Geometry check sheet. Reference: the model listing, model coordinates, mm. Face numbers are marked on the shaded views. A direction names the side the tool comes from. Coordinates: 2 decimals unless noted, no trailing zeros. Write each loop counter-clockwise with the first axis right and the second up, starting at its lowest first coordinate (ties: lowest second). Pieces come first, ordered by that corner, then holes. Notation, with made-up numbers: (32, 1) -> (67, 1) arc R23 ccw to (67, 27) -> close; hole circle Ø10 at (39.25, 41.5). An arc over 180 degrees is marked (long way). Answer in a Markdown table with one row per item. Add a question column.
1. Cross-section at A-A on y = 56.5. Record the cut outline in (x, z).
2. Cross-section at D-D on x = 14. Record the cut outline in (y, z).
3. Depth check by flat-ended pin: P1, Ø8, axis at y = 50, z = -22.5, coming from the +X side; P2, Ø1.5, axis at y = 59, z = -21.5, coming from the +X side; P3, Ø2.5, axis at y = 65.04, z = -23.5, coming from the +X side. Enter the tip coordinate at first touch or a pass-through.
4. Mould release check, pull along Y, two halves, no side actions. Record for the marked faces 1, 2 and 3: pulls with the +Y half, pulls with the -Y half, needs draft (parallel to the pull), parting line crosses it, or undercut.
5. Scan lines: L1, parallel to Y at x = 6.5, z = -29.5; L2, parallel to Y at x = 14, z = -20.25; L3, parallel to Y at x = 16.5, z = -29.75. Record each from-to range of solid material in increasing order. Write a range as from..to.
6. Set-up check for the marked faces 4, 5 and 6: record each of +Z, -Z, +X, -X, +Y, -Y from which the full face is reachable in a straight line by a thin tool's end or side.
7. Cross-section at C-C on z = -30.25. Record the cut outline in (x, y), and give its area (3 significant figures).
8. Cross-section at B-B on x = -9.5. Record the cut outline in (y, z).
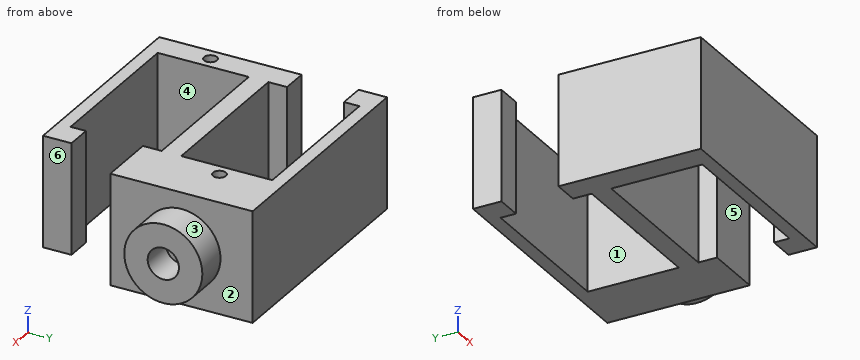
```python
from build123d import *

# Parameters (mm, degrees)
SKETCH2_W               = 32.000000477
SKETCH2_H               = 35
SKETCH2_W_2             = 22
SKETCH2_H_2             = 5
BOSS_EXTRUDE1_DEPTH     = 35
SKETCH3_W               = 15
SKETCH3_H               = 35
CUT_EXTRUDE1_DEPTH      = 90.56534365
CUT_EXTRUDE2_REACH      = 91.565
SKETCH4_W               = 20
SKETCH4_H               = 8.75
CUT_EXTRUDE3_REACH      = 91.565
SKETCH5_W               = 20
SKETCH5_H               = 8.75
SKETCH6_W               = 3
SKETCH6_H               = 35
CUT_EXTRUDE4_DEPTH      = 90.56534365
SKETCH11_R              = 1
CUT_EXTRUDE5_DEPTH      = 10
CUT_EXTRUDE6_DEPTH      = 80.508206961
CUT_EXTRUDE6_DEPTH_BACK = 17
CUT_EXTRUDE9_START      = -17
CUT_EXTRUDE9_DEPTH      = 17
SKETCH7_W               = 17
SKETCH7_H               = 21.875
BOSS_EXTRUDE2_DEPTH     = 5
SKETCH14_R              = 6
SKETCH14_R_2            = 2.4
BOSS_EXTRUDE6_DEPTH     = 5
CUT_EXTRUDE10_REACH     = 92.366
SKETCH15_R              = 1
SKETCH16_R              = 2
CUT_EXTRUDE11_DEPTH     = 7.000000238


# Read off the part's stored shape, not the designer's step: Cut-Extrude9
with BuildPart() as part:
    # Sketch2 → Boss-Extrude1 (new body)
    # profile 1 of 2: a face of its own
    with BuildSketch(Plane.XY):
        with Locations((0.112238017, 58.479936513)):
            Rectangle(SKETCH2_W, SKETCH2_H)
        Polygon((-10.887761984, 72.979936603), (-10.887761984, 43.979936513), (11.112238016, 43.979936513), (11.112238016, 72.979936513), align=None, mode=Mode.SUBTRACT)
    # profile 2 of 2: a face of its own
    with BuildSketch(Plane.XY):
        with Locations((0.112238016, 58.479936513)):
            Rectangle(SKETCH2_W_2, SKETCH2_H_2)
    extrude(amount=-BOSS_EXTRUDE1_DEPTH)

    # Sketch3 → Cut-Extrude1 (cut, through all)
    with BuildSketch(Plane(origin=(16.112238255, 0, 0), x_dir=(0, 0, -1), z_dir=(1, 0, 0))):
        with Locations((7.5, 58.479936513)):
            Rectangle(SKETCH3_W, SKETCH3_H)
    extrude(amount=-CUT_EXTRUDE1_DEPTH, mode=Mode.SUBTRACT)

    # Sketch4 → Cut-Extrude2 (cut, up to next)
    with BuildSketch(Plane.ZY.offset(15.887762222), mode=Mode.PRIVATE) as cut_extrude2_sk1:
        with Locations((-25, 67.229936513)):
            Rectangle(SKETCH4_W, SKETCH4_H)
    cut_extrude2_tool1 = extrude(cut_extrude2_sk1.sketch, amount=-CUT_EXTRUDE2_REACH, mode=Mode.PRIVATE) & part.part
    add(cut_extrude2_tool1.solids().sort_by_distance((-15.887762, 67.229937, -25))[0], mode=Mode.SUBTRACT)

    # Sketch5 → Cut-Extrude3 (cut, up to next)
    with BuildSketch(Plane(origin=(16.112238255, 0, 0), x_dir=(0, 0, -1), z_dir=(1, 0, 0)), mode=Mode.PRIVATE) as cut_extrude3_sk1:
        with Locations((25, 49.729936513)):
            Rectangle(SKETCH5_W, SKETCH5_H)
    cut_extrude3_tool1 = extrude(cut_extrude3_sk1.sketch, amount=-CUT_EXTRUDE3_REACH, mode=Mode.PRIVATE) & part.part
    add(cut_extrude3_tool1.solids().sort_by_distance((16.112238, 49.729937, -25))[0], mode=Mode.SUBTRACT)

    # Sketch6 → Cut-Extrude4 (cut, through all)
    with BuildSketch(Plane.ZY.offset(15.887762222)):
        with Locations((-33.5, 58.479936513)):
            Rectangle(SKETCH6_W, SKETCH6_H)
    extrude(amount=-CUT_EXTRUDE4_DEPTH, mode=Mode.SUBTRACT)

    # Sketch11 → Cut-Extrude5 (cut)
    with BuildSketch(Plane.XY.offset(-15)):
        with Locations((14.112238016, 66.979936513)):
            Circle(SKETCH11_R)
        with Locations((-13.887761984, 49.979936513)):
            Circle(SKETCH11_R)
    extrude(amount=-CUT_EXTRUDE5_DEPTH, mode=Mode.SUBTRACT)

    # Sketch12 → Cut-Extrude6 (cut, two sides: drawn at the far end of the back side and taken through both)
    with BuildSketch(Plane.XY.offset(-15).offset(-CUT_EXTRUDE6_DEPTH_BACK)):
        Polygon((-10.887761984, 62.854936513), (-11.887761984, 62.854936513), (-11.887761984, 59.979936513), (12.112238016, 59.979936513), (12.112238016, 73.979936509), (-11.887761984, 73.979936607), (-11.887761984, 71.604936513), (-10.887761984, 71.604936513), (-10.887761984, 72.979936603), (11.112238016, 72.979936513), (11.112238016, 60.979936513), (-10.887761984, 60.979936513), align=None)
    extrude(amount=CUT_EXTRUDE6_DEPTH + CUT_EXTRUDE6_DEPTH_BACK, mode=Mode.SUBTRACT)

    # Cut-Extrude9 outline → Cut-Extrude9 (cut)
    with BuildSketch(Plane.XY.offset(-15).offset(CUT_EXTRUDE9_START)):
        Polygon((12.112238016, 56.979936513), (-11.887761984, 56.979936513), (-11.887761984, 42.979936513), (12.112238016, 42.979936513), (12.112238016, 45.354936513), (11.112238016, 45.354936513), (11.112238016, 43.979936513), (-10.887761984, 43.979936513), (-10.887761984, 55.979936513), (11.112238016, 55.979936513), (11.112238016, 54.104936513), (12.112238016, 54.104936513), align=None)
    extrude(amount=CUT_EXTRUDE9_DEPTH, mode=Mode.SUBTRACT)

    # Sketch7 → Boss-Extrude2 (add)
    with BuildSketch(Plane(origin=(16.112238255, 0, 0), x_dir=(0, 0, -1), z_dir=(1, 0, 0))):
        with Locations((23.5, 65.042436513)):
            Rectangle(SKETCH7_W, SKETCH7_H)
    extrude(amount=BOSS_EXTRUDE2_DEPTH)

    # Sketch14 → Boss-Extrude6 (add)
    with BuildSketch(Plane(origin=(21.112238255, 0, 0), x_dir=(0, 0, -1), z_dir=(1, 0, 0))):
        with Locations(Location((23.5, 65.042436513, 0), (0, 0, 90))):
            Circle(SKETCH14_R)
        with Locations(Location((23.5, 65.042436513, 0), (0, 0, 90))):
            Circle(SKETCH14_R_2, mode=Mode.SUBTRACT)
    extrude(amount=BOSS_EXTRUDE6_DEPTH)

    # Sketch15 → Cut-Extrude10 (cut, up to next)
    with BuildSketch(Plane(origin=(21.112238255, 0, 0), x_dir=(0, 0, -1), z_dir=(1, 0, 0)), mode=Mode.PRIVATE) as cut_extrude10_sk1:
        with Locations(Location((23.5, 65.042436513, 0), (0, 0, 90))):
            Circle(SKETCH15_R)
    cut_extrude10_tool1 = extrude(cut_extrude10_sk1.sketch, amount=-CUT_EXTRUDE10_REACH, mode=Mode.PRIVATE) & part.part
    add(cut_extrude10_tool1.solids().sort_by_distance((21.112238, 65.042437, -23.5))[0], mode=Mode.SUBTRACT)

    # Sketch16 → Cut-Extrude11 (cut)
    with BuildSketch(Plane.ZY.offset(-12.112238016)):
        with Locations((-23.5, 65.042436513)):
            Circle(SKETCH16_R)
    extrude(amount=-CUT_EXTRUDE11_DEPTH, mode=Mode.SUBTRACT)


solid = part.part
```
Results found:
| question | item | result |
|---|---|---|
| 1 | outline | (-15.89, -32) -> (-11.89, -32) -> (-11.89, -15) -> (-15.89, -15) -> close; (12.11, -32) -> (21.11, -32) -> (21.11, -15) -> (12.11, -15) -> close |
| 2 | outline | (40.98, -32) -> (45.35, -32) -> (45.35, -15) -> (40.98, -15) -> close; (54.1, -32) -> (75.98, -32) -> (75.98, -15) -> (67.97, -15) -> (67.97, -25) -> (66.37, -25) arc R2 cw (long way) to (65.99, -21.74) -> (65.99, -15) -> (54.1, -15) -> close |
| 3 | P1 | stops at x = -11.89 |
| 3 | P2 | stops at x = 26.11 |
| 3 | P3 | stops at x = 21.11 |
| 4 | face 1 | undercut |
| 4 | face 2 | needs draft |
| 4 | face 3 | parting line crosses it |
| 5 | L1 | y = 40.98..42.98, 56.98..59.98, 73.98..75.98 |
| 5 | L2 | y = 40.98..45.35, 54.1..65.99, 67.97..75.98 |
| 5 | L3 | y = 54.1..75.98 |
| 6 | face 4 | +Z, -Z |
| 6 | face 5 | +Z, -Z, +X |
| 6 | face 6 | +Z, -Z, +X, -Y |
| 7 | outline | (-15.89, 40.98) -> (16.11, 40.98) -> (16.11, 45.35) -> (12.11, 45.35) -> (12.11, 42.98) -> (-11.89, 42.98) -> (-11.89, 56.98) -> (12.11, 56.98) -> (12.11, 54.1) -> (21.11, 54.1) -> (21.11, 75.98) -> (-15.89, 75.98) -> (-15.89, 71.6) -> (-11.89, 71.6) -> (-11.89, 73.98) -> (12.11, 73.98) -> (12.11, 59.98) -> (-11.89, 59.98) -> (-11.89, 62.85) -> (-15.89, 62.85) -> close |
| 7 | area | 487 mm^2 |
| 8 | outline | (40.98, -32) -> (42.98, -32) -> (42.98, -15) -> (40.98, -15) -> close; (56.98, -32) -> (59.98, -32) -> (59.98, -15) -> (56.98, -15) -> close; (73.98, -32) -> (75.98, -32) -> (75.98, -15) -> (73.98, -15) -> close |
